from build123d import *

# Parameters (mm, degrees)
SALIENTE_EXTRUIR1_DEPTH = 2


with BuildPart() as part:
    # Croquis1 → Saliente-Extruir1 (new body)
    with BuildSketch(Plane.XY):
        Polygon((0, 0), (0, -6), (-3, -6), (-3, -16), (0, -16), (0, -66), (-3, -66), (-3, -76), (0, -76), (0, -82), (28, -82), (28, -76), (31, -76), (31, -66), (28, -66), (28, -16), (31, -16), (31, -6), (28, -6), (28, 0), align=None)
    extrude(amount=-SALIENTE_EXTRUIR1_DEPTH)


solid = part.part
Read the model definition and answer for the solid it produces. Units are mm, in the model's axes. A direction names the side the tool comes from. Give positions to 0.01 mm unless a question says otherwise; leave off trailing zeros. Loops run counter-clockwise (first coordinate to the right, second up) from the corner with the lowest first, then second, coordinate; pieces in that order, holes last. Notation, with made-up numbers: (1.5, -3) -> (39.5, -3) arc R23 ccw to (39.5, 33) -> close; hole circle Ø10 at (46, 81.25). An arc over 180 degrees is marked (long way). Use a Markdown table: item, result.
Q1. Find the intervals of material crossed by line 1 along Y through (x, z) = (-1, -1.15); line 2 along X through (y, z) = (-42, -1.35), in increasing order.
Solved:
| item | result |
|---|---|
| line 1 | y = -76 to -66, -16 to -6 |
| line 2 | x = 0 to 28 |
Q2. A tool of negligible diameter and unlimited length cuts with its end or side. For faces 1 (the face through (-2, -76, -1)), 2 (the face through (-1, -6, -1)), 3 (the face through (-1, -66, -1)), from which of +Z, -Z, +X, -X, +Y, -Y can it reach the whole face along a straight path? Write none if from no direction.
Solved:
| item | result |
|---|---|
| face 1 | +Z, -Z, -X, -Y |
| face 2 | +Z, -Z, -X, +Y |
| face 3 | +Z, -Z, -X |
Q3. Section A-A, the plane z = -0.8 is taken. Determine the outline of the cut face in (x, y), then the cut area to 3 significant figures.
Solved:
| item | result |
|---|---|
| outline | (-3, -76) -> (0, -76) -> (0, -82) -> (28, -82) -> (28, -76) -> (31, -76) -> (31, -66) -> (28, -66) -> (28, -16) -> (31, -16) -> (31, -6) -> (28, -6) -> (28, 0) -> (0, 0) -> (0, -6) -> (-3, -6) -> (-3, -16) -> (0, -16) -> (0, -66) -> (-3, -66) -> close |
| area | 2,420 mm^2 |
Q4. Each of these flat-tipped pins is pushed along its axis until it touches: pin 1 (1 mm diameter, centred on x = -1.5, z = -0.5, fed in from -Y); pin 2 (1 mm diameter, centred on y = -79.5, z = -1, fed in from -X); pin 3 (1 mm diameter, centred on x = -2, z = -1, fed in from +Y). Where does it stop, or does it pass through?
Solved:
| item | result |
|---|---|
| pin 1 | stops at y = -76 |
| pin 2 | stops at x = 0 |
| pin 3 | stops at y = -6 |
Q5. Determine the mould class of faces 4 (the face through (30, -6, -1)), 5 (the face through (28, -79, -1)), 6 (the face through (29, -16, -1)) for opening direction Y: pulls with the +Y half, pulls with the -Y half, needs draft (parallel to the pull), parting line crosses it, or undercut.
Solved:
| item | result |
|---|---|
| face 4 | pulls with the +Y half |
| face 5 | needs draft |
| face 6 | undercut |
Q6. Section B-B, the plane y = -31.5 is taken. Determine the outline of the cut face in (x, z).
Solved:
| item | result |
|---|---|
| outline | (0, -2) -> (28, -2) -> (28, 0) -> (0, 0) -> close |
